Drawing for the job (mm, zero at the part's lowest x, y, z). Give positions to 0.01 mm unless a question says otherwise; leave off trailing zeros. Loops run counter-clockwise (first coordinate to the right, second up) from the corner with the lowest first, then second, coordinate; pieces in that order, holes last. Notation, with made-up numbers: (29.5, 83.25) -> (73.5, 83.25) arc R15 ccw to (73.5, 96.25) -> close; hole circle Ø1 at (58, 2). An arc over 180 degrees is marked (long way). Answer in a Markdown table with one row per item. Add a question column.
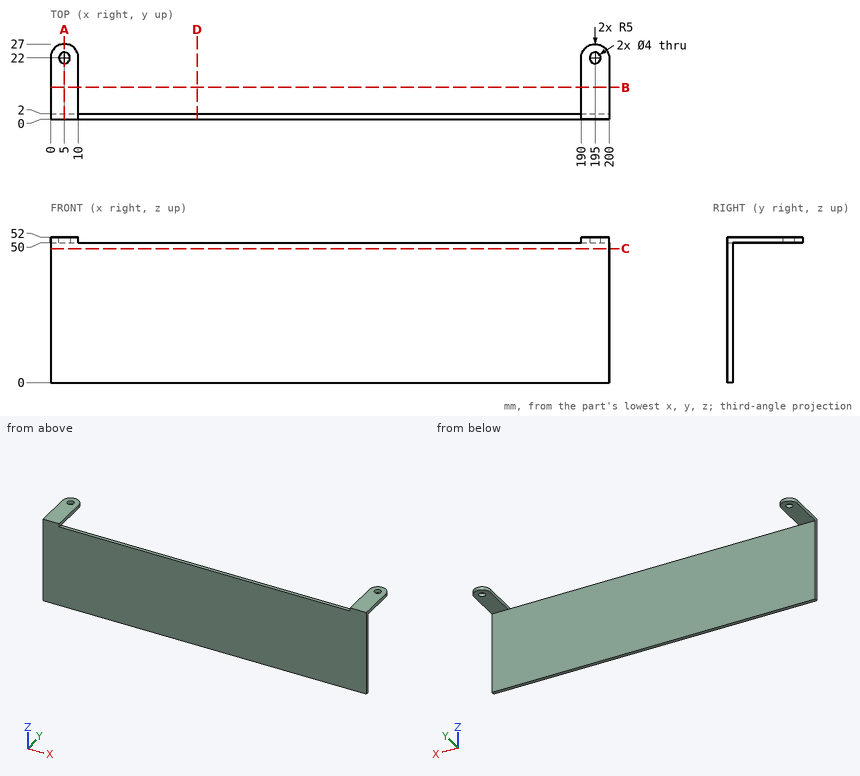
(1) Saw through at D-D, the plane x = 52.5. List the corners of the cut face in (y, z), then the cut area to 3 significant figures.
(2) Saw through at A-A, the plane x = 5. List the corners of the cut face in (y, z).
(3) Saw through at B-B, the plane y = 11.5. List the corners of the cut face in (x, z).
(4) Saw through at C-C, the plane z = 48. List the corners of the cut face in (x, y).
(5) Wall check: line 1 along Y through (x, z) = (122, 47.5); line 2 along Y through (x, z) = (195, 50.8); line 3 along Z through (x, y) = (151.5, 1). Give the ranges that are in metal, low to high. Write a range as from..to.
(6) Flat gauge pins, fed straight in: pin 1 Ø15 at (x, z) = (55, 24) entering from +Y; pin 2 Ø8 at (x, y) = (6.5, 13.5) entering from -Z; pin 3 Ø1 at (x, y) = (139.5, 1) entering from +Z. Where does each tip first touch, or does it go through?
Worked answers:
| question | item | result |
|---|---|---|
| 1 | outline | (0, 0) -> (2, 0) -> (2, 50) -> (0, 50) -> close |
| 1 | area | 100 mm^2 |
| 2 | outline | (0, 0) -> (2, 0) -> (2, 50) -> (20, 50) -> (20, 52) -> (0, 52) -> close; (24, 50) -> (27, 50) -> (27, 52) -> (24, 52) -> close |
| 3 | outline | (0, 50) -> (10, 50) -> (10, 52) -> (0, 52) -> close; (190, 50) -> (200, 50) -> (200, 52) -> (190, 52) -> close |
| 4 | outline | (0, 0) -> (200, 0) -> (200, 2) -> (0, 2) -> close |
| 5 | line 1 | 0..2 |
| 5 | line 2 | 0..20, 24..27 |
| 5 | line 3 | 0..50 |
| 6 | pin 1 | y = 2 |
| 6 | pin 2 | z = 50 |
| 6 | pin 3 | z = 50 |
